Geometry: final body of the model. Coordinates: model frame, mm. Face numbers are marked on the shaded views. A direction names the side the tool comes from. Round coordinates to 2 decimals unless told otherwise and drop trailing zeros. Loops run counter-clockwise (first coordinate to the right, second up) from the corner with the lowest first, then second, coordinate; pieces in that order, holes last. Notation, with made-up numbers: M 79.5,27 L 121.5,27 A17 ccw 121.5,37 Z; hole C -35.75,-28 d8. An arc over 180 degrees is marked long. Answer as a JSON object with one key per item and string values.
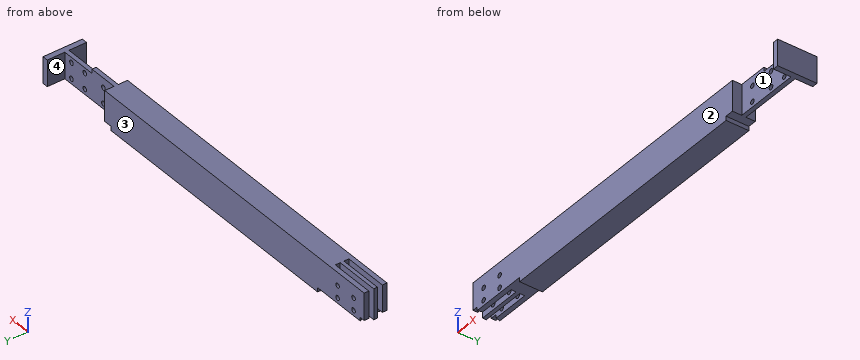
from build123d import *

# Parameters (mm, degrees)
SKETCH1_W                  = 1176
SKETCH1_H                  = 75
BOSS_EXTRUDE1_DEPTH        = 65
SKETCH2_W                  = 776
SKETCH2_H                  = 65
BOSS_EXTRUDE2_DEPTH        = 12
SKETCH3_W                  = 1058
SKETCH3_H                  = 65
BOSS_EXTRUDE3_DEPTH        = 12
SKETCH4_W                  = 16
SKETCH4_H                  = 23.5
SKETCH4_H_2                = 65
BOSS_EXTRUDE4_DEPTH        = 75
CUT_EXTRUDE1_DEPTH         = 601.953617179
CUT_EXTRUDE1_DEPTH_BACK    = 601.953617179
SKETCH5_W                  = 102
SKETCH5_H                  = 50
F_12_0MM_DOWEL_HOLE1_D     = 13.5
F_12_0MM_DOWEL_HOLE1_DEPTH = 65
CUT_EXTRUDE2_DEPTH         = 10
CUT_EXTRUDE3_DEPTH         = 601.953617179
CUT_EXTRUDE3_DEPTH_BACK    = 601.953617179
SKETCH11_W                 = 127.490852802
SKETCH11_H                 = 14
CUT_EXTRUDE4_DEPTH         = 601.953617179
CUT_EXTRUDE4_DEPTH_BACK    = 601.953617179
SKETCH12_W                 = 83
SKETCH12_H                 = 26.5


with BuildPart() as part:
    # Sketch1 → Boss-Extrude1 (new body)
    with BuildSketch(Plane(origin=(0, 0, 0), x_dir=(1, 0, 0), z_dir=(0, 1, 0))):
        Rectangle(SKETCH1_W, SKETCH1_H)
    extrude(amount=BOSS_EXTRUDE1_DEPTH)

    # Sketch2 → Boss-Extrude2 (add)
    with BuildSketch(Plane.XY.offset(-37.5)):
        with Locations((-25, 32.5)):
            Rectangle(SKETCH2_W, SKETCH2_H)
    extrude(amount=-BOSS_EXTRUDE2_DEPTH)

    # Sketch3 → Boss-Extrude3 (add)
    with BuildSketch(Plane.XY.offset(37.5)):
        with Locations((-59, 32.5)):
            Rectangle(SKETCH3_W, SKETCH3_H)
    extrude(amount=BOSS_EXTRUDE3_DEPTH)

    # Sketch4 → Boss-Extrude4 (add)
    with BuildSketch(Plane.XY.offset(37.5)):
        with Locations((580, -11.75)):
            Rectangle(SKETCH4_W, SKETCH4_H)
        with Locations((580, 32.5)):
            Rectangle(SKETCH4_W, SKETCH4_H_2)
        with Locations((580, 76.75)):
            Rectangle(SKETCH4_W, SKETCH4_H)
    extrude(amount=-BOSS_EXTRUDE4_DEPTH)

    # Sketch5 → Cut-Extrude1 (cut, two sides: drawn at the far end of the back side and taken through both)
    with BuildSketch(Plane.XY.offset(37.5).offset(-CUT_EXTRUDE1_DEPTH_BACK)):
        with Locations((521, 1.5)):
            Rectangle(SKETCH5_W, SKETCH5_H)
        with Locations((521, 63.5)):
            Rectangle(SKETCH5_W, SKETCH5_H)
    extrude(amount=CUT_EXTRUDE1_DEPTH + CUT_EXTRUDE1_DEPTH_BACK, mode=Mode.SUBTRACT)

    # Ø12.0mm Dowel Hole1
    with Locations(Plane(origin=(0, 65, 0), x_dir=(1, 0, 0), z_dir=(0, 1, 0))):
        with Locations((-548, -12.5), (-488, -12.5), (-488, 22.5), (-548, 22.5), (427, 22.5), (497, 22.5), (547, 22.5), (547, -22.5), (497, -22.5), (427, -22.5)):
            Hole(F_12_0MM_DOWEL_HOLE1_D / 2, depth=F_12_0MM_DOWEL_HOLE1_DEPTH)

    # Sketch9 → Cut-Extrude2 (cut)
    with BuildSketch(Plane(origin=(0, 0, -37.5), x_dir=(-1, 0, 0), z_dir=(0, 0, -1))):
        with BuildLine():
            Line((462, 51.75), (462, 37.75))
            Line((462, 37.75), (600.472295571, 37.75))
            ThreePointArc((600.472295571, 37.75), (600.253164472, 32.5), (600.472295571, 27.25))
            Line((600.472295571, 27.25), (462, 27.25))
            Line((462, 27.25), (462, 13.25))
            Line((462, 13.25), (569.202978401, 13.25))
            ThreePointArc((569.202978401, 13.25), (759.253164472, 32.5), (569.202978401, 51.75))
            Line((569.202978401, 51.75), (462, 51.75))
        make_face()
    extrude(amount=-CUT_EXTRUDE2_DEPTH, mode=Mode.SUBTRACT)

    # Sketch11 → Cut-Extrude3 (cut, two sides: drawn at the far end of the back side and taken through both)
    with BuildSketch(Plane(origin=(0, 0, -37.5), x_dir=(-1, 0, 0), z_dir=(0, 0, -1)).offset(-CUT_EXTRUDE3_DEPTH_BACK)):
        with Locations((525.745426401, 44.75)):
            Rectangle(SKETCH11_W, SKETCH11_H)
        with Locations((525.745426401, 20.25)):
            Rectangle(SKETCH11_W, SKETCH11_H)
    extrude(amount=CUT_EXTRUDE3_DEPTH + CUT_EXTRUDE3_DEPTH_BACK, mode=Mode.SUBTRACT)

    # Sketch12 → Cut-Extrude4 (cut, two sides: drawn at the far end of the back side and taken through both)
    with BuildSketch(Plane(origin=(0, 0, -37.5), x_dir=(-1, 0, 0), z_dir=(0, 0, -1)).offset(-CUT_EXTRUDE4_DEPTH_BACK)):
        with Locations((-428.5, 13.25)):
            Rectangle(SKETCH12_W, SKETCH12_H)
        with Locations((-428.5, 51.75)):
            Rectangle(SKETCH12_W, SKETCH12_H)
    extrude(amount=CUT_EXTRUDE4_DEPTH + CUT_EXTRUDE4_DEPTH_BACK, mode=Mode.SUBTRACT)


solid = part.part
1) Pin query (flat end, axial travel): P1, Ø15.5, axis at x = -488, z = 12.5, coming from the +Y side; P2, Ø15.5, axis at x = -548, z = 12.5, coming from the -Y side; P3, Ø3, axis at y = 69.5, z = -0.5, coming from the -X side. Return the tip coordinate at first contact, or that it passes through.
Results:
{"P1": "y = 65", "P2": "y = 0", "P3": "x = 572"}
2) Reachability of the marked faces 1, 2, 3 and 4 from +Z, -Z, +X, -X, +Y, -Y: full face, straight path, thin tool, end or side. Return the list, or none.
Results:
{"face 1": "+Z, -Z, -Y", "face 2": "+Z, -Z, -X, -Y", "face 3": "+Z, -Z, -X, +Y", "face 4": "+Z, -Z, +Y"}
3) Ray query, line 1 (X direction, y = 6, z = 12); line 2 (Z direction, x = 497, y = 33.25); line 3 (Z direction, x = -488, y = 59). Return the intervals inside material, ascending.
Results:
{"line 1": "-588 to -554.73, -541.27 to -494.73, -481.27 to 387, 572 to 588", "line 2": "-37.5 to -29.25, -15.75 to 15.75, 29.25 to 37.5", "line 3": "-37.5 to -29.25, -15.75 to 5.75, 19.25 to 49.5"}
4) Section query A-A (x = -242.5). Return the cut outline in (y, z), and give its area (4 significant figures).
Results:
{"outline": "M 0,-49.5 L 65,-49.5 L 65,49.5 L 0,49.5 Z", "area": "6,435 mm2"}
